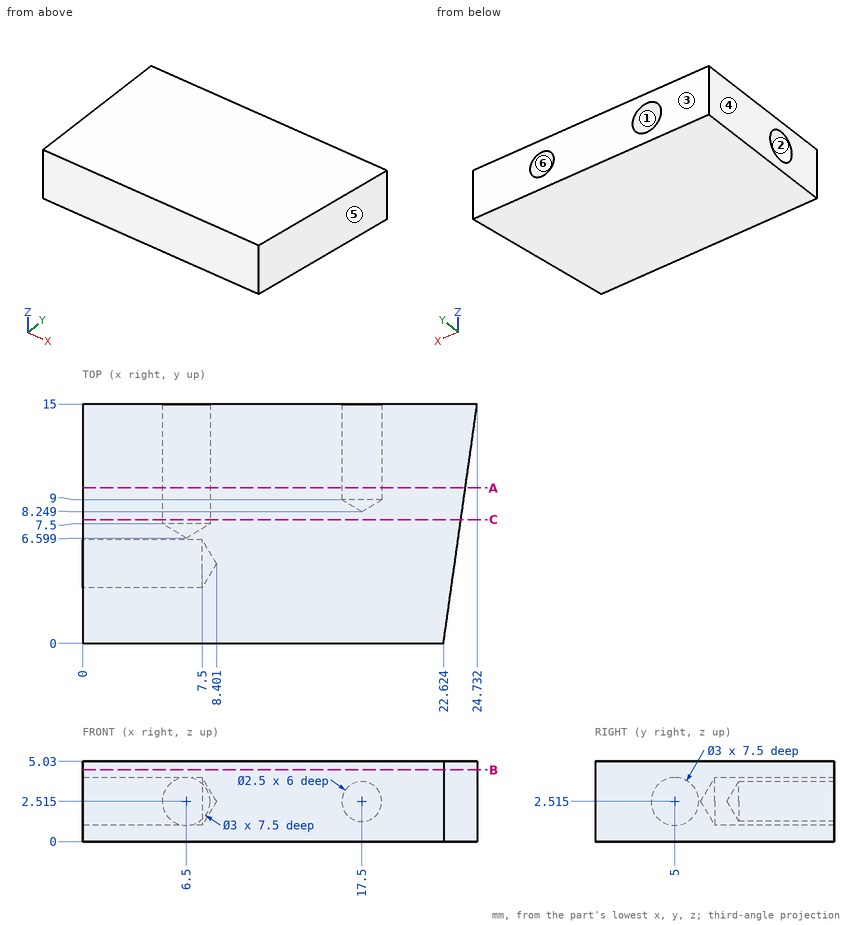
Verification items for this drawing (mm, ordinates from the low corner). A direction names the side the tool comes from. Round coordinates to 2 decimals unless told otherwise and drop trailing zeros. Order: outer loops, then holes, each group sorted by start corner. A loop starts at its lowest first (then second) coordinate and runs counter-clockwise, first axis right, second up. Notation, with made-up numbers: (73.25, 45.25) - (87.25, 45.25) arc R16 cw to (87.25, 50.25) - close; hole circle Ø10 at (-17, -2.5). An arc over 180 degrees is marked (long way). Use CSV: the item, a comma, the result in double quotes. Start each with the question number.
1) Mould release check, pull along X, two halves, no side actions. Record for the marked faces 4, 5 and 6: +X half, -X half, draft (parallel to the pull), parting line (faces both ways), or undercut.
2) Access from +Z, -Z, +X, -X, +Y, -Y to the whole of each face (thin tool, end or side, straight path). Record for the marked faces 1, 2 and 3.
3) Thickness scan on L1, parallel to Z at x = 4.75, y = 5 (1 decimal); L2, parallel to X at y = 14.25, z = 2.85 (1 decimal); L3, parallel to Z at x = 17.5, y = 12 (1 decimal). Record the ranges inside material, lowest first.
4) Section check B-B, the plane z = 4.5. Record the cut outline in (x, y) (1 decimal), plus the area to 3 significant figures.
5) Go/stop test with flat-tipped pins: P1, Ø3, axis at x = 18.5, z = 2, coming from the +Y side; P2, Ø1.8, axis at y = 5, z = 2.515, coming from the -X side. Record where each tip stops, or that it passes through.
6) Section check A-A, the plane y = 9.75. State how many separate pieces and enclosed holes the cut face has, plus the area to 3 significant figures.
7) Section check C-C, the plane y = 7.75. Record the cut outline in (x, z) (1 decimal), plus the area to 3 significant figures.
Answers:
1,face 4,"-X half"
1,face 5,"+X half"
1,face 6,"undercut"
2,face 1,"+Y"
2,face 2,"-X"
2,face 3,"+Z, -Z, +X, -X, +Y"
3,L1,"z = 0 to 1, 4 to 5"
3,L2,"x = 0 to 5, 8 to 16.3, 18.7 to 24.6"
3,L3,"z = 0 to 1.3, 3.8 to 5"
4,outline,"(0, 0) - (22.6, 0) - (24.7, 15) - (0, 15) - close"
4,area,"355 mm²"
5,P1,"stops at y = 15"
5,P2,"stops at x = 7.86"
6,separate pieces,"1"
6,enclosed holes,"2"
6,area,"109 mm²"
7,outline,"(0, 0) - (23.7, 0) - (23.7, 5) - (0, 5) - close; hole circle Ø3 at (6.5, 2.5)"
7,area,"112 mm²"
